```python
from build123d import *

# Parameters (mm, degrees)
ESQUISSE2_OUTSIDE_W   = 92.28
ESQUISSE2_OUTSIDE_H   = 92.28
ESQUISSE2_OUTSIDE_W_2 = 10
ESQUISSE2_OUTSIDE_H_2 = 24.610755802
EXTRUSION1_DEPTH      = 10


with BuildPart() as part:
    # Esquisse1 → Révolution1 (revolve)
    with BuildSketch(Plane.XY):
        Polygon((0, 0), (8, 0), (8, 60), (8.45, 60), (8.45, 69.4), (9, 69.4), (9, 74.4), (8.45, 74.4), (8.45, 85.5), (8.5, 85.5), (8.5, 95.5), (8.45, 95.5), (8.45, 348), (8.5, 348), (8.5, 358.4), (7.75, 358.4), (7.75, 359.5), (8.45, 359.5), (8.45, 360.5), (0, 360.5), align=None)
    revolve(axis=Axis((0, 0, 0), (0, 1, 0)))

    # Esquisse2 outside → Extrusion1 (cut)
    with BuildSketch(Plane.XZ):
        Rectangle(ESQUISSE2_OUTSIDE_W, ESQUISSE2_OUTSIDE_H)
        Rectangle(ESQUISSE2_OUTSIDE_W_2, ESQUISSE2_OUTSIDE_H_2, mode=Mode.SUBTRACT)
    extrude(amount=-EXTRUSION1_DEPTH, mode=Mode.SUBTRACT)


solid = part.part
```
Model file for the job. Use its own axes, mm. A direction names the side the tool comes from. Coordinates: 2 decimals unless noted, no trailing zeros. Loops run counter-clockwise (first coordinate to the right, second up) from the corner with the lowest first, then second, coordinate; pieces in that order, holes last. Notation, with made-up numbers: (-38.5, 66.5) - (18.5, 66.5) arc R22 cw to (18.5, 85.5) - close; hole circle Ø9 at (-24.5, 66.5). An arc over 180 degrees is marked (long way). Write item = value, one per line. Start each with the question number.
Item 1: Pull direction Y, two halves, no side cores. Call faces 1 (the face through (-1.009, 358.958, -7.684)), 2 (the face through (8, 358.4, -2)), 3 (the face through (0, 0, 0)), 4 (the face through (4.57, 353.273, -7.167)): +Y half, -Y half, draft (parallel to the pull), parting line (faces both ways), or undercut.
Item 2: Wall check: probe 1 along Y at (x, z) = (-6, -5.5); probe 2 along X at (y, z) = (54, 0.5); probe 3 along Z at (x, y) = (-3.25, 108). Give the ranges that are in metal, low to high. Write a range as [from, to].
Item 3: Saw through at A-A, the plane y = 330. List the corners of the cut face in (x, z), then the cut area to 3 significant figures.
Item 4: Drop flat-ended pins along their axis: pin 1 Ø0.9 at (x, z) = (6.5, -1) entering from -Y; pin 2 Ø6 at (y, z) = (152.5, -1.5) entering from +X; pin 3 Ø3 at (y, z) = (115, 2.5) entering from -X. Give the stop position or say it passes through.
Item 5: 3-axis set-ups, long thin cutter, end or side, ignore diameter. For faces 5 (the face through (4.57, 90.57, -7.167)), 6 (the face through (-5, 5, 0)), 7 (the face through (-7, 69.4, 5)): which of +Z, -Z, +X, -X, +Y, -Y reach the whole face in a straight line?
Answers:
q1.face_1 = undercut
q1.face_2 = undercut
q1.face_3 = -Y half
q1.face_4 = draft
q2.probe_1 = [60, 358.4], [359.5, 360.5]
q2.probe_2 = [-7.98, 7.98]
q2.probe_3 = [-7.8, 7.8]
q3.outline = circle Ø16.9 at (0, 0)
q3.area = 224 mm2
q4.pin_1 = 10
q4.pin_2 = 8.45
q4.pin_3 = -8.39
q5.face_5 = +Y
q5.face_6 = +Z, -Z, -X, -Y
q5.face_7 = -Y
